For this review, take the finished solid that the model builds, in its own axes (mm). Round coordinates to 2 decimals unless told otherwise and drop trailing zeros. Write each loop counter-clockwise with the first axis right and the second up, starting at its lowest first coordinate (ties: lowest second). Pieces come first, ordered by that corner, then holes.
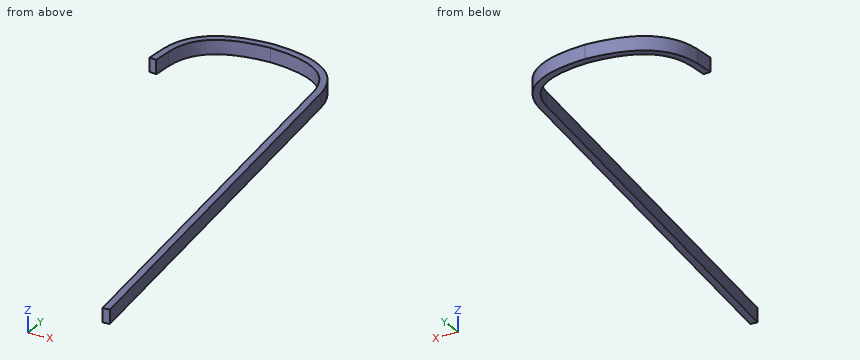
from build123d import *

# Parameters (mm, degrees)
BOSS_EXTRUDE1_DEPTH = 19.05


with BuildPart() as part:
    # Sketch1 → Boss-Extrude1 (new body)
    with BuildSketch(Plane.XY):
        with BuildLine():
            Line((154.716315659, 154.51789158), (97.403993572, 735.828587024))
            add(Edge.make_bspline(
                [(0, 803.26908628), (0.979817658, 803.233925105), (2.950075123, 803.151909058), (6.800362849, 802.946009068), (11.504912112, 802.608232022), (16.957304332, 802.075979486), (23.975792063, 801.198424891), (32.273128008, 799.790052384), (41.46699497, 797.614109593), (49.89784204, 794.967332344), (60.129456963, 790.832450746), (71.050790712, 784.572420078), (79.648241417, 776.932392043), (85.274313562, 769.943199813), (88.89525226, 764.228265264), (91.933130485, 758.00316425), (93.979934001, 752.359286407), (95.321414001, 747.554999291), (96.177362738, 743.805316844), (96.764020616, 740.553537606), (97.155379667, 737.881968465), (97.326205951, 736.51096636), (97.403993572, 735.828587024)],
                knots=[0.000508173, 0.000508173, 0.000508173, 0.000508173, 0.016098161, 0.031688149, 0.062868125, 0.094048101, 0.125228077, 0.187588029, 0.249947981, 0.312307933, 0.374667885, 0.499387789, 0.624107693, 0.686467645, 0.748827597, 0.811187549, 0.873547501, 0.904727477, 0.935907453, 0.967087429, 0.982677417, 0.998267405, 0.998267405, 0.998267405, 0.998267405], degree=3))
            add(Edge.make_bspline(
                [(-97.403993572, 735.828587024), (-97.326205951, 736.51096636), (-97.155379667, 737.881968465), (-96.764020616, 740.553537606), (-96.177362738, 743.805316844), (-95.321414001, 747.554999291), (-93.979934001, 752.359286407), (-91.933130485, 758.00316425), (-88.89525226, 764.228265264), (-85.274313562, 769.943199813), (-79.648241417, 776.932392043), (-71.050790712, 784.572420078), (-60.129456963, 790.832450746), (-49.89784204, 794.967332344), (-41.46699497, 797.614109593), (-32.273128008, 799.790052384), (-23.975792063, 801.198424891), (-16.957304332, 802.075979486), (-11.504912112, 802.608232022), (-6.800362849, 802.946009068), (-2.950075123, 803.151909058), (-0.979817658, 803.233925105), (0, 803.26908628)],
                knots=[0.000508173, 0.000508173, 0.000508173, 0.000508173, 0.016098161, 0.031688149, 0.062868125, 0.094048101, 0.125228077, 0.187588029, 0.249947981, 0.312307933, 0.374667885, 0.499387789, 0.624107693, 0.686467645, 0.748827597, 0.811187549, 0.873547501, 0.904727477, 0.935907453, 0.967087429, 0.982677417, 0.998267405, 0.998267405, 0.998267405, 0.998267405], degree=3))
            Line((-97.403993572, 735.828587024), (-99.889181424, 710.621681669))
            Line((-99.889181424, 710.621681669), (-109.368223301, 711.556235093))
            Line((-109.368223301, 711.556235093), (-106.876080835, 736.833680097))
            add(Edge.make_bspline(
                [(-106.876080835, 736.833680097), (-98.655564568, 809.385111394), (0, 812.8)],
                knots=[0, 0, 0, 1, 1, 1], degree=2))
            add(Edge.make_bspline(
                [(106.876080835, 736.833680097), (98.655564568, 809.385111394), (0, 812.8)],
                knots=[0, 0, 0, 1, 1, 1], degree=2))
            Line((106.876080835, 736.833680097), (164.195357535, 155.452445004))
            Line((164.195357535, 155.452445004), (154.716315659, 154.51789158))
        make_face()
    extrude(amount=BOSS_EXTRUDE1_DEPTH)


solid = part.part
(1) For line 1 along X through (y, z) = (712.5, 2.5); line 2 along X through (y, z) = (761, 1.25); line 3 along X through (y, z) = (553.5, 8), list the stretches that pass through material, from the lowest coordinate up.
Geometry check:
line 1: x = -109.28 to -99.7, 99.7 to 109.28
line 2: x = -100.87 to -90.44, 90.44 to 100.87
line 3: x = 115.38 to 124.95
(2) We need section B-B, the plane y = 275.5. Give the boundary of the cut face in (x, z), and give its area (3 significant figures).
Geometry check:
outline: (142.79, 0) - (152.36, 0) - (152.36, 19.05) - (142.79, 19.05) - close
area: 182 mm2
(3) We need section A-A, the plane x = 126. Give the boundary of the cut face in (y, z), and give its area (3 significant figures).
Geometry check:
outline: (445.78, 0) - (542.86, 0) - (542.86, 19.05) - (445.78, 19.05) - close
area: 1,850 mm2
(4) For pin 1 Ø8 at (x, z) = (-38, 16) entering from +Y; pin 2 Ø3 at (y, z) = (476, 4) entering from +X; pin 3 Ø4 at (x, z) = (-69.5, 5) entering from +Y, all flat-tipped, find the tip position at first contact; note any pin that passes through.
Geometry check:
pin 1: stops at y = 809.05
pin 2: stops at x = 132.74
pin 3: stops at y = 797.42
